from build123d import *

# Parameters (mm, degrees)
SKETCH1_W           = 18
SKETCH1_H           = 4
BOSS_EXTRUDE1_DEPTH = 5
SKETCH2_R           = 7
BOSS_EXTRUDE2_DEPTH = 15
SKETCH3_R           = 6
CUT_EXTRUDE1_DEPTH  = 21
CUT_EXTRUDE2_DEPTH  = 4


with BuildPart() as part:
    # Sketch1 → Boss-Extrude1 (new body)
    with BuildSketch(Plane(origin=(0, 0, 0), x_dir=(1, 0, 0), z_dir=(0, 1, 0))):
        with Locations((0, 7)):
            Rectangle(SKETCH1_W, SKETCH1_H)
        with Locations((0, -7)):
            Rectangle(SKETCH1_W, SKETCH1_H)
        with BuildLine():
            Line((-9, -5), (9, -5))
            ThreePointArc((9, -5), (14, 0), (9, 5))
            Line((9, 5), (-9, 5))
            ThreePointArc((-9, 5), (-14, 0), (-9, -5))
        make_face()
    extrude(amount=BOSS_EXTRUDE1_DEPTH)

    # Sketch2 → Boss-Extrude2 (add)
    with BuildSketch(Plane(origin=(0, 5, 0), x_dir=(1, 0, 0), z_dir=(0, 1, 0))):
        Circle(SKETCH2_R)
    extrude(amount=BOSS_EXTRUDE2_DEPTH)

    # Sketch3 → Cut-Extrude1 (cut, through all)
    with BuildSketch(Plane(origin=(0, 20, 0), x_dir=(1, 0, 0), z_dir=(0, 1, 0))):
        Circle(SKETCH3_R)
    extrude(amount=-CUT_EXTRUDE1_DEPTH, mode=Mode.SUBTRACT)

    # Sketch4 → Cut-Extrude2 (cut)
    with BuildSketch(Plane.XZ):
        with BuildLine():
            Line((8, -8), (8, -3.872983346))
            ThreePointArc((8, -3.872983346), (13, 0), (8, 3.872983346))
            Line((8, 3.872983346), (8, 8))
            Line((8, 8), (-8, 8))
            Line((-8, 8), (-8, 3.872983346))
            ThreePointArc((-8, 3.872983346), (-13, 0), (-8, -3.872983346))
            Line((-8, -3.872983346), (-8, -8))
            Line((-8, -8), (8, -8))
        make_face()
    extrude(amount=-CUT_EXTRUDE2_DEPTH, mode=Mode.SUBTRACT)


solid = part.part
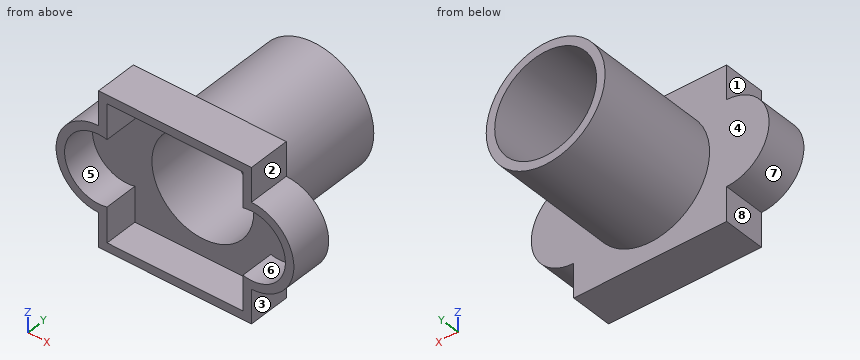
Check sheet for the modelled part. Datum: model origin and axes. Units: mm. Face numbers are marked on the shaded views. A direction names the side the tool comes from. Coordinates: 2 decimals unless noted, no trailing zeros. Loops run counter-clockwise (first coordinate to the right, second up) from the corner with the lowest first, then second, coordinate; pieces in that order, holes last. Notation, with made-up numbers: (11, 70) -> (43, 70) arc R20 ccw to (43, 97) -> close; hole circle Ø2 at (-8.5, 72.5). An arc over 180 degrees is marked (long way). Write item = value, one per line. Start each with the question number.
1. Tool access check on the marked faces 1, 2, 3, 4 and 5. Record the directions out of +Z, -Z, +X, -X, +Y, -Y that give a thin tool (end or side, any length) a straight path to the whole face; none if there is none.
2. Section check A-A on z = 0. Record the cut outline in (x, y).
3. Draft check along Z on the marked faces 6, 7 and 8. Enter one of: released by +Z, released by -Z, zero draft, split by the parting line, or undercut.
4. Section check C-C on x = -1. Record the cut outline in (y, z).
5. Depth check by flat-ended pin: P1, Ø1.2, axis at y = 3.5, z = 7.5, coming from the +X side; P2, Ø1.5, axis at y = 6.5, z = -4, coming from the +X side; P3, Ø4, axis at x = 2.5, y = 11.5, coming from the -Z side. Enter the tip coordinate at first touch or a pass-through.
6. Section check D-D on z = -7.5. Record the cut outline in (x, y).
7. Material ranges on line 1 (X direction, y = 3, z = -6.25); line 2 (X direction, y = 14.25, z = 0); line 3 (Z direction, x = -0.25, y = 19.25), recorded low to high.
8. Section check B-B on y = 2. Record the cut outline in (x, z).
Responses:
q1.face_1 = +Z, -X, +Y, -Y
q1.face_2 = +Z, +X, +Y, -Y
q1.face_3 = -Z, +X, +Y, -Y
q1.face_4 = +Y
q1.face_5 = -Y
q2.outline = (-14, 0) -> (-13, 0) -> (-13, 4) -> (-6, 4) -> (-6, 20) -> (-7, 20) -> (-7, 5) -> (-14, 5) -> close; (6, 4) -> (13, 4) -> (13, 0) -> (14, 0) -> (14, 5) -> (7, 5) -> (7, 20) -> (6, 20) -> close
q3.face_6 = undercut
q3.face_7 = split by the parting line
q3.face_8 = zero draft
q4.outline = (0, -9) -> (5, -9) -> (5, -6.93) -> (20, -6.93) -> (20, -5.92) -> (4, -5.92) -> (4, -8) -> (0, -8) -> close; (0, 8) -> (4, 8) -> (4, 5.92) -> (20, 5.92) -> (20, 6.93) -> (5, 6.93) -> (5, 9) -> (0, 9) -> close
q5.P1 = 9
q5.P2 = 6.2
q5.P3 = -6.98
q6.outline = (-9, 0) -> (-8, 0) -> (-8, 4) -> (8, 4) -> (8, 0) -> (9, 0) -> (9, 5) -> (-9, 5) -> close
q7.line_1 = -9 to -8, 8 to 9
q7.line_2 = -7 to -6, 6 to 7
q7.line_3 = -7 to -5.99, 5.99 to 7
q8.outline = (-9, -9) -> (9, -9) -> (9, -5) arc R5 ccw to (9, 5) -> (9, 9) -> (-9, 9) -> (-9, 5) arc R5 ccw to (-9, -5) -> close; hole (-8, -8) -> (8, -8) -> (8, -3.87) arc R4 ccw (long way) to (8, 3.87) -> (8, 8) -> (-8, 8) -> (-8, 3.87) arc R4 ccw (long way) to (-8, -3.87) -> close
